Geometry: final body of the model. Coordinates: model frame, mm. A direction names the side the tool comes from. Give positions to 0.01 mm unless a question says otherwise; leave off trailing zeros. Write each loop counter-clockwise with the first axis right and the second up, starting at its lowest first coordinate (ties: lowest second). Pieces come first, ordered by that corner, then holes.
Q1. Line query: L1, parallel to Y at x = 0, z = 5.25; L2, parallel to Y at x = 5, z = 6.5; L3, parallel to X at y = 0, z = 8.5. Output: solid intervals per line, ascending.
Q2. Cut plane A-A on x = 0. Return the cut outline in (y, z), plus the area to 3 significant figures.
Q3. Cut plane B-B on y = 0. Return the cut outline in (x, z), plus the area to 3 significant figures.
Q4. Cut plane D-D on z = 4.75. Return the cut outline in (x, y).
Q5. Pin query (flat end, axial travel): pin 1 (3 mm diameter, centred on x = -34, y = -9.5, fed in from +Z). Return the tip coordinate at first contact, or that it passes through.
Q6. Draft query along X for faces 1 (the face through (35.04, -0.36, 10.12)), 2 (the face through (38.1, 0, 6)), 3 (the face through (-1, 25.4, 6)). Return one class per face: pulls with the +X half, pulls with the -X half, needs draft (parallel to the pull), parting line crosses it, or undercut.
Q7. Cut plane C-C on z = 11.75. Return the cut outline in (x, y).
Q8. Reachability of faces 4 (the face through (-5.186, -18, 11)), 5 (the face through (30, 0, 7.62)), 6 (the face through (8, 12, 0)) from +Z, -Z, +X, -X, +Y, -Y: full face, straight path, thin tool, end or side. Return the list, or none.
```python
from build123d import *

# Parameters (mm, degrees)
F0_W     = 76.2
F0_H     = 50.8
F0_R     = 12.7
F1_DEPTH = 12.7
F2_W     = 6.35
F2_H     = 50.8
F3_DEPTH = 2.54
F5_DEPTH = 50.8


with BuildPart() as f1:
    # F0 (on Top) → F1 (new body)
    with BuildSketch(Plane.XY):
        Rectangle(F0_W, F0_H)
        Circle(F0_R, mode=Mode.SUBTRACT)
    extrude(amount=F1_DEPTH)

    # F2 (on face) → F3 (cut)
    with BuildSketch(Plane.XY.offset(12.7)):
        with BuildLine():
            Line((-5.1856809296, -11.5930459025), (-5.1856809296, -25.4))
            Line((-5.1856809296, -25.4), (4.9743190704, -25.4))
            Line((4.9743190704, -25.4), (4.9743190704, -11.6852963071))
            ThreePointArc((4.9743190704, -11.6852963071), (-0.1153082528, -12.6994765249), (-5.1856809296, -11.5930459025))
        make_face()
        with BuildLine():
            Line((4.9743190704, 25.4), (-5.1856809296, 25.4))
            Line((-5.1856809296, 25.4), (-5.1856809296, 11.5930459025))
            ThreePointArc((-5.1856809296, 11.5930459025), (-0.1153082528, 12.6994765249), (4.9743190704, 11.6852963071))
            Line((4.9743190704, 11.6852963071), (4.9743190704, 25.4))
        make_face()
        with Locations((-32.385, 0)):
            Rectangle(F2_W, F2_H)
    extrude(amount=-F3_DEPTH, mode=Mode.SUBTRACT)

    # F4 (on face) → F5 (cut, through all)
    with BuildSketch(Plane.XZ.offset(25.4)):
        Polygon((33.5493190704, 12.7), (27.1993190704, 12.7), (24.2663797029, 7.62), (36.4822584379, 7.62), align=None)
    extrude(amount=-F5_DEPTH, mode=Mode.SUBTRACT)


solid = f1.part
```
Data:
1. L1: y = -25.4 to -12.7, 12.7 to 25.4
1. L2: y = -25.4 to -11.67, 11.67 to 25.4
1. L3: x = -38.1 to -12.7, 12.7 to 24.77, 35.97 to 38.1
2. outline: (-25.4, 0) - (-12.7, 0) - (-12.7, 10.16) - (-25.4, 10.16) - close; (12.7, 0) - (25.4, 0) - (25.4, 10.16) - (12.7, 10.16) - close
2. area: 258 mm2
3. outline: (-38.1, 0) - (-12.7, 0) - (-12.7, 12.7) - (-29.21, 12.7) - (-29.21, 10.16) - (-35.56, 10.16) - (-35.56, 12.7) - (-38.1, 12.7) - close; (12.7, 0) - (38.1, 0) - (38.1, 12.7) - (33.55, 12.7) - (36.48, 7.62) - (24.27, 7.62) - (27.2, 12.7) - (12.7, 12.7) - close
3. area: 582 mm2
4. outline: (-38.1, -25.4) - (38.1, -25.4) - (38.1, 25.4) - (-38.1, 25.4) - close; hole circle Ø25.4 at (0, 0)
5. pin 1: stops at z = 10.16
6. face 1: undercut
6. face 2: pulls with the +X half
6. face 3: needs draft
7. outline: (-38.1, -25.4) - (-35.56, -25.4) - (-35.56, 25.4) - (-38.1, 25.4) - close; (-29.21, -25.4) - (-5.19, -25.4) - (-5.19, -11.59) arc R12.7 cw to (-5.19, 11.59) - (-5.19, 25.4) - (-29.21, 25.4) - close; (4.97, -25.4) - (26.65, -25.4) - (26.65, 25.4) - (4.97, 25.4) - (4.97, 11.69) arc R12.7 cw to (4.97, -11.69) - close; (34.1, -25.4) - (38.1, -25.4) - (38.1, 25.4) - (34.1, 25.4) - close
8. face 4: +Z, +Y, -Y
8. face 5: +Y, -Y
8. face 6: -Z, +X, -X, +Y, -Y
